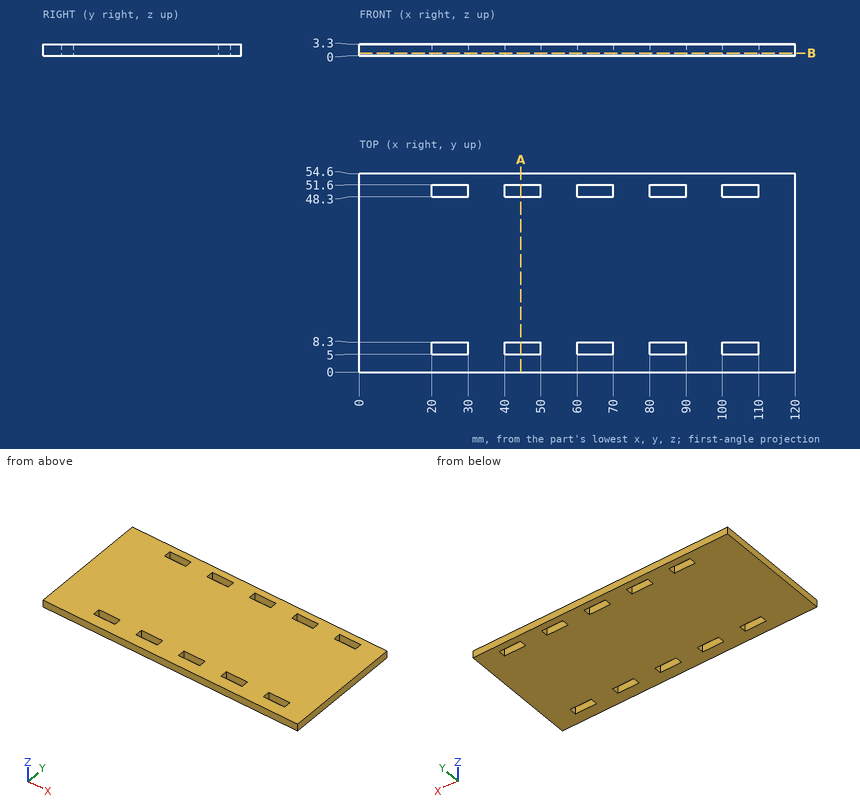
Design review of the part shown in the three views and the two pictorial views. Dimensions are in mm from the part's minimum x, y and z. Round coordinates to 2 decimals unless told otherwise and drop trailing zeros. Order: outer loops, then holes, each group sorted by start corner. A loop starts at its lowest first (then second) coordinate and runs counter-clockwise, first axis right, second up. Notation, with made-up numbers: (69, 49.5) -> (105, 49.5) arc R25 ccw to (105, 86.5) -> close; hole circle Ø2 at (-20, 45). An arc over 180 degrees is marked (long way). Write item = value, one per line. Start each with the question number.
1) Take a section at B-B on z = 0.8. Count the separate pieces of the cut face and the enclosed holes in it, plus the area to 3 significant figures.
2) Insertion check: pin 1 (1 mm diameter, centred on x = 42, y = 45.5, fed in from -Z). The pin has a flat end and moves straight along its axis. Give the tip position at first contact, or say it passes through.
3) Take a section at A-A on x = 44.5. State the section outline as (y, z) points, plus the area to 3 significant figures.
4) To check wall thickness, follow line 1 (X direction, y = 8, z = 2.65); line 2 (Y direction, x = 41, z = 2.4). State the ranges of each line that lie inside material, in increasing order. Write a range as from..to.
Verdict:
q1.separate_pieces = 1
q1.enclosed_holes = 10
q1.area = 6,220 mm2
q2.pin_1 = 0
q3.outline = (0, 0) -> (5, 0) -> (5, 3.3) -> (0, 3.3) -> close; (8.3, 0) -> (48.3, 0) -> (48.3, 3.3) -> (8.3, 3.3) -> close; (51.6, 0) -> (54.6, 0) -> (54.6, 3.3) -> (51.6, 3.3) -> close
q3.area = 158 mm2
q4.line_1 = 0..20, 30..40, 50..60, 70..80, 90..100, 110..120
q4.line_2 = 0..5, 8.3..48.3, 51.6..54.6
